Can you work these out from the drawing? Everything is in mm from the part's minimum corner. Round coordinates to 2 decimals unless told otherwise and drop trailing zeros. Write each loop counter-clockwise with the first axis right and the second up, starting at its lowest first coordinate (ties: lowest second). Pieces come first, ordered by that corner, then holes. Notation, with made-up numbers: (85.5, -36) -> (106.5, -36) arc R28 ccw to (106.5, -15) -> close; hole circle Ø8 at (35.25, 0.25). An arc over 180 degrees is marked (long way). Write item = value, one per line. Start each with the question number.
1) Imagine slicing it at A-A, the plane y = 2.25. Please give me the cut outline in (x, z).
2) If I drill on line 1 (Z direction, x = 0.35, y = 2.4); line 2 (X direction, y = 2.4, z = 23.5); line 3 (X direction, y = 1.5, z = 35), over which ranges is the centre line in solid material (lowest first)?
3) Thinking about a two-plate mould opening in Z: for the marked faces 1, 2 and 3, which applies, +Z half, -Z half, draft (parallel to the pull), parting line (faces both ways), or undercut?
4) Imagine slicing it at C-C, the plane z = 23.5. Please give me the cut outline in (x, y), then the cut area to 3 significant figures.
5) I'm going to push a flat-ended pin straight in: pin 1 (1 mm diameter, centred on y = 1.5, z = 25.5, fed in from -X). Where does the tip first touch, or does it pass through?
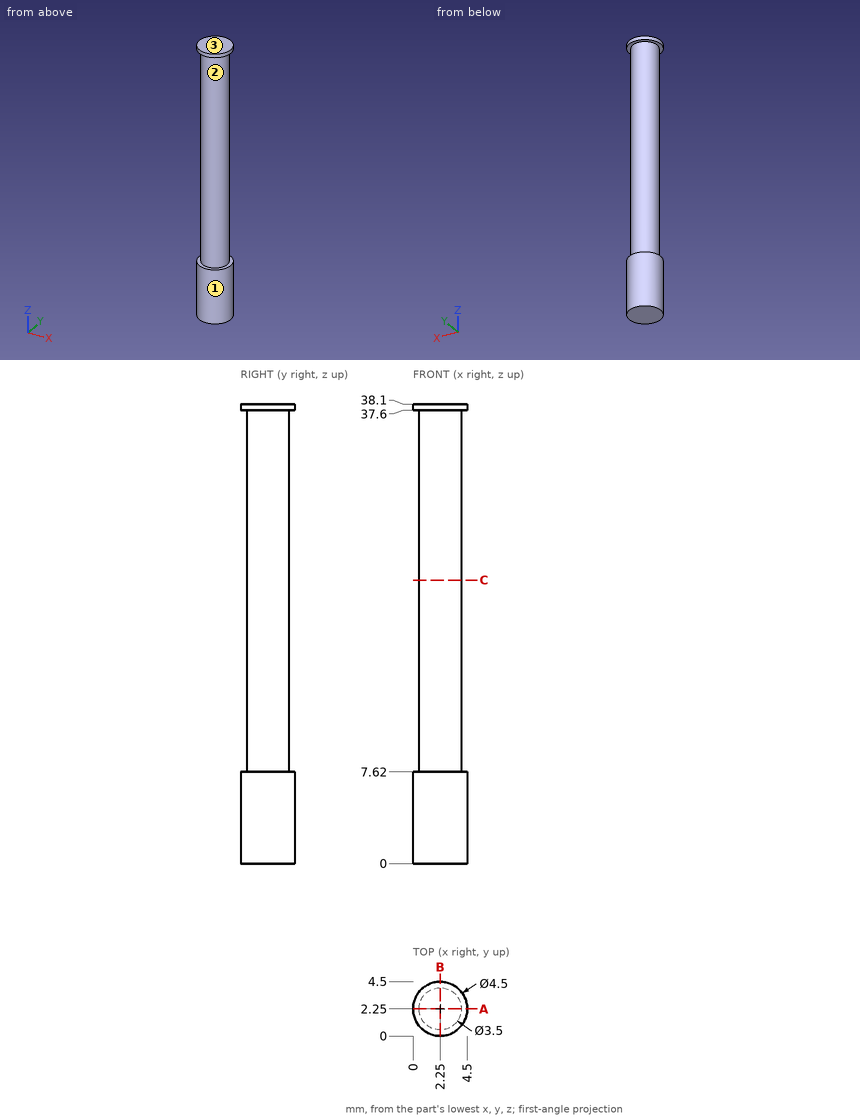
Reported:
q1.outline = (0, 0) -> (4.5, 0) -> (4.5, 7.62) -> (4, 7.62) -> (4, 37.6) -> (4.5, 37.6) -> (4.5, 38.1) -> (0, 38.1) -> (0, 37.6) -> (0.5, 37.6) -> (0.5, 7.62) -> (0, 7.62) -> close
q2.line_1 = 0 to 7.62, 37.6 to 38.1
q2.line_2 = 0.51 to 3.99
q2.line_3 = 0.67 to 3.83
q3.face_1 = draft
q3.face_2 = undercut
q3.face_3 = +Z half
q4.outline = circle Ø3.5 at (2.25, 2.25)
q4.area = 9.62 mm²
q5.pin_1 = 0.52
